from build123d import *
from build123d.topology import SkipClean

# Parameters (mm, degrees)
SKETCH2_W            = 35
SKETCH2_H            = 55
BOSS_EXTRUDE1_DEPTH  = 45
BOSS_EXTRUDE2_DEPTH  = 5
SKETCH6_R            = 17.5
BOSS_EXTRUDE3_DEPTH  = 12
BOSS_EXTRUDE4_START  = 5
BOSS_EXTRUDE4_DEPTH  = 5
BOSS_EXTRUDE5_START  = 12
SKETCH8_R            = 17.5
BOSS_EXTRUDE5_DEPTH  = 12
BOSS_EXTRUDE6_START  = -12
BOSS_EXTRUDE6_DEPTH  = 12
BOSS_EXTRUDE7_DEPTH  = 12
SKETCH14_W           = 24.5
SKETCH14_H           = 45.4
CUT_EXTRUDE3_DEPTH   = 12
SKETCH15_R           = 21.1
CUT_EXTRUDE4_DEPTH   = 12
CUT_EXTRUDE5_DEPTH   = 139.069755203
SKETCH21_R           = 1.25
CUT_EXTRUDE7_DEPTH   = 12
SKETCH23_R           = 10.1
BOSS_EXTRUDE8_DEPTH  = 6
SKETCH24_R           = 8.5
CUT_EXTRUDE8_DEPTH   = 6
SKETCH25_R           = 2.7
CUT_EXTRUDE9_DEPTH   = 18
BOSS_EXTRUDE9_START  = -12
BOSS_EXTRUDE9_DEPTH  = 12
SKETCH30_R           = 1.25
CUT_EXTRUDE11_DEPTH  = 12
SKETCH31_R           = 2
CUT_EXTRUDE12_DEPTH  = 2.5
BOSS_EXTRUDE11_DEPTH = 12


with BuildPart() as part:
    # Sketch2 → Boss-Extrude1 (new body)
    with BuildSketch(Plane.XY):
        with BuildLine():
            ThreePointArc((-17.5, 27.5), (0, 45), (17.5, 27.5))
            Line((17.5, 27.5), (-17.5, 27.5))
        make_face()
        Rectangle(SKETCH2_W, SKETCH2_H)
        with BuildLine():
            ThreePointArc((17.5, -27.5), (0, -45), (-17.5, -27.5))
            Line((-17.5, -27.5), (17.5, -27.5))
        make_face()
    extrude(amount=BOSS_EXTRUDE1_DEPTH)

    # Sketch5 → Boss-Extrude2 (add)
    with SkipClean():  # the faces are left unmerged after this step: merging them gives an invalid solid
        with BuildSketch(Plane.XY.offset(45)):
            with BuildLine():
                ThreePointArc((17.5, 27.5), (0, 45), (-17.5, 27.5))
                ThreePointArc((-17.5, 27.5), (0, 10), (17.5, 27.5))
            make_face()
        extrude(amount=BOSS_EXTRUDE2_DEPTH)

    # Sketch6 → Boss-Extrude3 (add)
    with BuildSketch(Plane.XY.offset(50)):
        with BuildLine():
            Line((-17.5, 67.5), (17.5, 67.5))
            ThreePointArc((17.5, 67.5), (0, 85), (-17.5, 67.5))
        make_face()
        with BuildLine():
            Line((17.5, 27.5), (17.5, 67.5))
            Line((17.5, 67.5), (-17.5, 67.5))
            Line((-17.5, 67.5), (-17.5, 27.5))
            ThreePointArc((-17.5, 27.5), (0, 45), (17.5, 27.5))
        make_face()
        with Locations(Location((0, 27.5, 0), (0, 0, 180))):
            Circle(SKETCH6_R)
    extrude(amount=BOSS_EXTRUDE3_DEPTH)

    # Sketch7 → Boss-Extrude4 (add)
    with SkipClean():  # the faces are left unmerged after this step: merging them gives an invalid solid
        with BuildSketch(Plane(origin=(0, 0, 0), x_dir=(-1, 0, 0), z_dir=(0, 0, -1)).offset(BOSS_EXTRUDE4_START)):
            with BuildLine():
                ThreePointArc((17.5, 27.5), (0, 10), (-17.5, 27.5))
                ThreePointArc((-17.5, 27.5), (0, 45), (17.5, 27.5))
            make_face()
        extrude(amount=-BOSS_EXTRUDE4_DEPTH)
    add(part.part.scale(1), mode=Mode.REPLACE)  # the faces are merged on a copy

    # Sketch8 → Boss-Extrude5 (add)
    with SkipClean():  # the faces are left unmerged after this step: merging them gives an invalid solid
        with BuildSketch(Plane(origin=(0, 0, -5), x_dir=(-1, 0, 0), z_dir=(0, 0, -1)).offset(BOSS_EXTRUDE5_START)):
            with BuildLine():
                Line((17.5, 67.5), (-17.5, 67.5))
                ThreePointArc((-17.5, 67.5), (0, 85), (17.5, 67.5))
            make_face()
            with BuildLine():
                ThreePointArc((-17.5, 27.5), (0, 45), (17.5, 27.5))
                Line((17.5, 27.5), (17.5, 67.5))
                Line((17.5, 67.5), (-17.5, 67.5))
                Line((-17.5, 67.5), (-17.5, 27.5))
            make_face()
            with Locations((0, 27.5)):
                Circle(SKETCH8_R)
        extrude(amount=-BOSS_EXTRUDE5_DEPTH)

    # Sketch11 → Boss-Extrude6 (add)
    with BuildSketch(Plane.XY.offset(62).offset(BOSS_EXTRUDE6_START)):
        with BuildLine():
            Line((-17.5, 67.5), (-17.5, 27.5))
            ThreePointArc((-17.5, 27.5), (0, 10), (17.5, 27.5))
            Line((17.5, 27.5), (17.5, 67.5))
            ThreePointArc((17.5, 67.5), (0, 115.060885195), (-17.5, 67.5))
        make_face()
    extrude(amount=BOSS_EXTRUDE6_DEPTH)

    # Sketch12 → Boss-Extrude7 (add)
    with BuildSketch(Plane(origin=(0, 0, -17), x_dir=(-1, 0, 0), z_dir=(0, 0, -1))):
        with BuildLine():
            ThreePointArc((17.5, 67.5), (0, 115.060885195), (-17.5, 67.5))
            ThreePointArc((-17.5, 67.5), (0, 85), (17.5, 67.5))
        make_face()
    extrude(amount=-BOSS_EXTRUDE7_DEPTH)

    # Sketch14 → Cut-Extrude3 (cut)
    with BuildSketch(Plane.XY.offset(62)):
        with Locations((0, 77.710885195)):
            Rectangle(SKETCH14_W, SKETCH14_H)
    extrude(amount=-CUT_EXTRUDE3_DEPTH, mode=Mode.SUBTRACT)

    # Sketch15 → Cut-Extrude4 (cut)
    with BuildSketch(Plane(origin=(0, 0, -17), x_dir=(-1, 0, 0), z_dir=(0, 0, -1))):
        with Locations((0, 88.060885195)):
            Circle(SKETCH15_R)
    extrude(amount=-CUT_EXTRUDE4_DEPTH, mode=Mode.SUBTRACT)

    # Sketch17 → Cut-Extrude5 (cut, through all)
    with BuildSketch(Plane.ZY.offset(17.5)):
        Polygon((10, -27.5), (22.5, -27.5), (35, -27.5), (35, -15.5), (10, -15.5), align=None)
        Polygon((35, -27.5), (22.5, -27.5), (10, -27.5), (10, -45), (35, -45), align=None)
    extrude(amount=-CUT_EXTRUDE5_DEPTH, mode=Mode.SUBTRACT)

    # Sketch21 → Cut-Extrude7 (cut)
    with BuildSketch(Plane.XY.offset(45)):
        with Locations((8, -27.5)):
            Circle(SKETCH21_R)
        with Locations((5.656854249, -33.156854249)):
            Circle(SKETCH21_R)
        with Locations((0, -35.5)):
            Circle(SKETCH21_R)
        with Locations((-5.656854249, -33.156854249)):
            Circle(SKETCH21_R)
        with Locations((-8, -27.5)):
            Circle(SKETCH21_R)
        with Locations((-5.656854249, -21.843145751)):
            Circle(SKETCH21_R)
        with Locations((0, -19.5)):
            Circle(SKETCH21_R)
        with Locations((5.656854249, -21.843145751)):
            Circle(SKETCH21_R)
    extrude(amount=-CUT_EXTRUDE7_DEPTH, mode=Mode.SUBTRACT)

    # Sketch23 → Boss-Extrude8 (add)
    with BuildSketch(Plane(origin=(0, 0, 0), x_dir=(-1, 0, 0), z_dir=(0, 0, -1))):
        with Locations(Location((0, -27.5, 0), (0, 0, 180))):
            Circle(SKETCH23_R)
    extrude(amount=BOSS_EXTRUDE8_DEPTH)

    # Sketch24 → Cut-Extrude8 (cut)
    with BuildSketch(Plane(origin=(0, 0, -6), x_dir=(-1, 0, 0), z_dir=(0, 0, -1))):
        with Locations((0, -27.5)):
            Circle(SKETCH24_R)
    extrude(amount=-CUT_EXTRUDE8_DEPTH, mode=Mode.SUBTRACT)

    # Sketch25 → Cut-Extrude9 (cut)
    with BuildSketch(Plane(origin=(0, 0, 0), x_dir=(-1, 0, 0), z_dir=(0, 0, -1))):
        with Locations((0, -27.5)):
            Circle(SKETCH25_R)
    extrude(amount=-CUT_EXTRUDE9_DEPTH, mode=Mode.SUBTRACT)

    # Sketch26 → Boss-Extrude9 (add)
    with BuildSketch(Plane.XY.offset(62).offset(BOSS_EXTRUDE9_START)):
        with BuildLine():
            ThreePointArc((-17.5, 67.5), (-23.313699367, 74.442095901), (-26.505269682, 82.915918813))
            ThreePointArc((-26.505269682, 82.915918813), (-22.976087169, 55.049770191), (-17.5, 27.5))
            Line((-17.5, 27.5), (-17.5, 67.5))
        make_face()
        with BuildLine():
            ThreePointArc((17.5, 27.5), (22.976087169, 55.049770191), (26.505269682, 82.915918813))
            ThreePointArc((26.505269682, 82.915918813), (23.313699367, 74.442095901), (17.5, 67.5))
            Line((17.5, 67.5), (17.5, 27.5))
        make_face()
    extrude(amount=BOSS_EXTRUDE9_DEPTH)

    # Sketch30 → Cut-Extrude11 (cut)
    with BuildSketch(Plane.XY.offset(62)):
        with Locations((15, 92.910885195)):
            Circle(SKETCH30_R)
        with Locations((15, 75.910885195)):
            Circle(SKETCH30_R)
        with Locations((15, 58.910885195)):
            Circle(SKETCH30_R)
        with Locations(Location((-15, 92.910885195, 0), (0, 0, 180))):
            Circle(SKETCH30_R)
        with Locations(Location((-15, 75.910885195, 0), (0, 0, 180))):
            Circle(SKETCH30_R)
        with Locations(Location((-15, 58.910885195, 0), (0, 0, 180))):
            Circle(SKETCH30_R)
    extrude(amount=-CUT_EXTRUDE11_DEPTH, mode=Mode.SUBTRACT)

    # Sketch31 → Cut-Extrude12 (cut)
    with BuildSketch(Plane(origin=(0, 0, 50), x_dir=(-1, 0, 0), z_dir=(0, 0, -1))):
        with Locations((15, 92.910885195)):
            Circle(SKETCH31_R)
        with Locations((15, 75.910885195)):
            Circle(SKETCH31_R)
        with Locations((15, 58.910885195)):
            Circle(SKETCH31_R)
        with Locations(Location((-15, 58.910885195, 0), (0, 0, 180))):
            Circle(SKETCH31_R)
        with Locations(Location((-15, 75.910885195, 0), (0, 0, 180))):
            Circle(SKETCH31_R)
        with Locations(Location((-15, 92.910885195, 0), (0, 0, 180))):
            Circle(SKETCH31_R)
    extrude(amount=-CUT_EXTRUDE12_DEPTH, mode=Mode.SUBTRACT)

    # Sketch32 → Boss-Extrude11 (add)
    with BuildSketch(Plane(origin=(0, 0, -17), x_dir=(-1, 0, 0), z_dir=(0, 0, -1))):
        with BuildLine():
            ThreePointArc((-17.5, 67.5), (-23.313699367, 74.442095901), (-26.505269682, 82.915918813))
            ThreePointArc((-26.505269682, 82.915918813), (-22.976087169, 55.049770191), (-17.5, 27.5))
            Line((-17.5, 27.5), (-17.5, 67.5))
        make_face()
        with BuildLine():
            ThreePointArc((17.5, 27.5), (22.976087169, 55.049770191), (26.505269682, 82.915918813))
            ThreePointArc((26.505269682, 82.915918813), (23.313699367, 74.442095901), (17.5, 67.5))
            Line((17.5, 67.5), (17.5, 27.5))
        make_face()
    extrude(amount=-BOSS_EXTRUDE11_DEPTH)


solid = part.part
The listing builds one solid part. Answer for the finished solid, in the listing's coordinates (mm). A direction names the side the tool comes from. Coordinates: 2 decimals unless noted, no trailing zeros. Write each loop counter-clockwise with the first axis right and the second up, starting at its lowest first coordinate (ties: lowest second). Pieces come first, ordered by that corner, then holes. Notation, with made-up numbers: M -20.75,-7.75 L 16.25,-7.75 A24 cw 16.25,25.25 Z; hole C 71.25,83.5 d6. An arc over 180 degrees is marked long. Write each question's results on one line, items separated by ' | '.
Item 1: The part is cut by section C-C on y = 50.5. Determine the outline of the cut face in (x, z), and give its area (3 significant figures).
Answer below:
outline: M -22.21,-17 L 22.21,-17 L 22.21,-5 L -22.21,-5 Z; M -22.21,50 L 22.21,50 L 22.21,62 L -22.21,62 Z | area: 1,070 mm2
Item 2: Which of the six approach directions +Z, -Z, +X, -X, +Y, -Y give full straight-line access (tool end or side, diameter ignored) to faces 4 (the face through (12.25, 77, 56)), 5 (the face through (4, -30, 10)), 6 (the face through (14.566, 77.863, 51.232)), 7 (the face through (1.84, -35.8, -3.04))?
Answer below:
face 4: +Z | face 5: +X, -X, -Y | face 6: none | face 7: -Z
Item 3: The part is cut by section A-A on z = 55.5. Determine the outline of the cut face in (x, y).
Answer below:
outline: M -26.51,82.92 A400 ccw -17.5,27.5 A17.5 ccw 17.5,27.5 A400 ccw 26.51,82.92 A27 ccw long Z; hole C -15,58.91 d2.5; hole C -15,75.91 d2.5; hole C -15,92.91 d2.5; hole M -12.25,55.01 L 12.25,55.01 L 12.25,100.41 L -12.25,100.41 Z; hole C 15,58.91 d2.5; hole C 15,75.91 d2.5; hole C 15,92.91 d2.5
Item 4: The part is cut by section B-B on y = 97.5. Determine the outline of the cut face in (x, z), and give its area (3 significant figures).
Answer below:
outline: M -25.3,-17 L -18.87,-17 L -18.87,-5 L -25.3,-5 Z; M -25.3,50 L -12.25,50 L -12.25,62 L -25.3,62 Z; M 12.25,50 L 25.3,50 L 25.3,62 L 12.25,62 Z; M 18.87,-17 L 25.3,-17 L 25.3,-5 L 18.87,-5 Z | area: 467 mm2
Item 5: Given P1, Ø6, axis at y = 64.5, z = -1, coming from the +X side; P2, Ø4.5, axis at x = -15, y = 92.91, coming from the -Z side; P3, Ø1, axis at x = 9.5, z = 23.5, coming from the -Y side; P4, Ø10, axis at x = -12.5, z = 43.5, coming from the +Y side, each flat-ended and moving along its own axis, determine where each tip first touches the part or whether it passes through.
Answer below:
P1: through | P2: z = 50 | P3: y = -15.5 | P4: y = 43.31
Item 6: Consider probe 1 along Z at (x, y) = (12.5, 62.5); probe 2 along X at (y, z) = (-27, 39); probe 3 along Z at (x, y) = (14, -21.5). Determine where each line is inside the solid, lowest interval first. Write a range as [from, to].
Answer below:
probe 1: [-17, -5], [50, 62] | probe 2: [-17.5, -9.15], [-6.85, 6.85], [9.15, 17.5] | probe 3: [0, 10], [35, 45]
Item 7: For a pull along X with two mould halves and no side action, classify faces 1 (the face through (-22.913, 54.662, -11.084)), 2 (the face through (0, -30, 35)), 3 (the face through (-14.566, 73.958, 51.232)) as released by +X, released by -X, zero draft, split by the parting line, or undercut.
Answer below:
face 1: released by -X | face 2: zero draft | face 3: undercut
Item 8: The part is cut by section D-D on z = -8. Determine the outline of the cut face in (x, y), and give its area (3 significant figures).
Answer below:
outline: M -26.51,82.92 A400 ccw -17.5,27.5 A17.5 ccw 17.5,27.5 A400 ccw 26.51,82.92 A27 ccw long Z; hole C 0,88.06 d42.2 | area: 3,020 mm2
